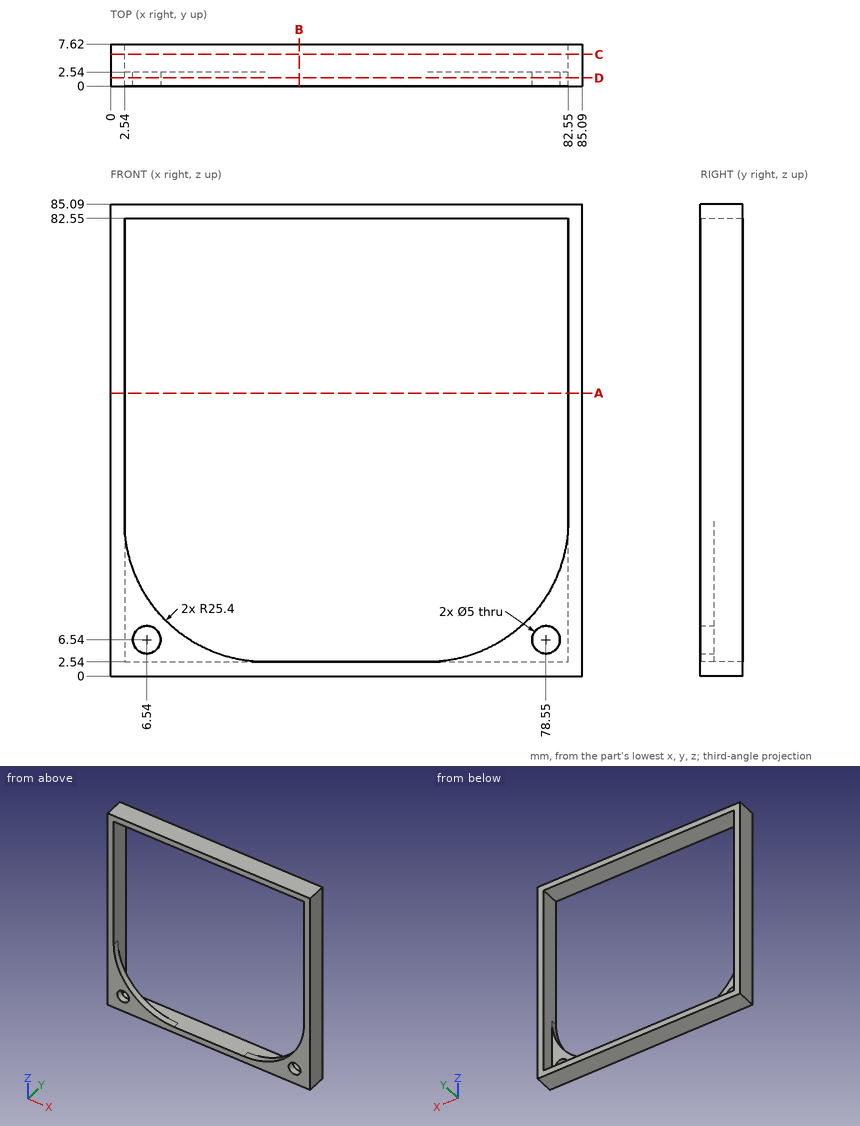
Design review of the part shown in the three views and the two pictorial views. Dimensions are in mm from the part's minimum x, y and z. Give positions to 0.01 mm unless a question says otherwise; leave off trailing zeros. Loops run counter-clockwise (first coordinate to the right, second up) from the corner with the lowest first, then second, coordinate; pieces in that order, holes last. Notation, with made-up numbers: (-5.75, 87.5) -> (39.25, 87.5) arc R26 ccw to (39.25, 111.5) -> close; hole circle Ø8 at (41, 63.5). An arc over 180 degrees is marked (long way). Answer as a JSON object with one key per item and string values. Group by question number.
Q1. Take a section at C-C (y = 5.75). Write out the cut boundary in (x, z), plus the area to 3 significant figures.
Q2. Wall thickness on line 1 along Z through (x, y) = (19.5, 4.75); line 2 along X through (y, z) = (1.4, 6.54): over which ranges is each line inside the solid? List them lowest first.
Q3. Take a section at D-D (y = 1.5). Write out the cut boundary in (x, z), plus the area to 3 significant figures.
Q4. Take a section at A-A (z = 51). Write out the cut boundary in (x, y).
Q5. Take a section at B-B (x = 34). Write out the cut boundary in (y, z), plus the area to 3 significant figures.
Answer below:
{
 "1": {"outline": "(0, 0) -> (85.09, 0) -> (85.09, 85.09) -> (0, 85.09) -> close; hole (2.54, 2.54) -> (82.55, 2.54) -> (82.55, 82.55) -> (2.54, 82.55) -> close", "area": "839 mm2"},
 "2": {"line 1": "z = 0 to 2.54, 82.55 to 85.09", "line 2": "x = 0 to 4.04, 9.04 to 14.26, 70.83 to 76.05, 81.05 to 85.09"},
 "3": {"outline": "(0, 0) -> (85.09, 0) -> (85.09, 85.09) -> (0, 85.09) -> close; hole (2.54, 27.94) arc R25.4 ccw to (27.94, 2.54) -> (57.15, 2.54) arc R25.4 ccw to (82.55, 27.94) -> (82.55, 82.55) -> (2.54, 82.55) -> close; hole circle Ø5 at (6.54, 6.54); hole circle Ø5 at (78.55, 6.54)", "area": "1,080 mm2"},
 "4": {"outline": "(0, 0) -> (2.54, 0) -> (2.54, 7.62) -> (0, 7.62) -> close; (82.55, 0) -> (85.09, 0) -> (85.09, 7.62) -> (82.55, 7.62) -> close"},
 "5": {"outline": "(0, 0) -> (7.62, 0) -> (7.62, 2.54) -> (0, 2.54) -> close; (0, 82.55) -> (7.62, 82.55) -> (7.62, 85.09) -> (0, 85.09) -> close", "area": "38.7 mm2"}
}
